Autodesk Inventor part; units mm, degrees
ref_plane "YZ Plane" through (0, 0, 0) normal (1, 0, 0) x (0, 1, 0)
ref_plane "XZ Plane" through (0, 0, 0) normal (0, 1, 0) x (-1, 0, 0)
ref_plane "XY Plane" through (0, 0, 0) normal (0, 0, 1) x (1, 0, 0)
sketch "Sketch1" plane through (0, 0, 0) normal (1, 0, 0) x (0, 1, 0)
  line L0 (9.0933, 11.7239) -> (-29.0067, 11.7239)
  line L1 (-29.0067, 11.7239) -> (-29.0067, -26.3761)
  line L2 (-29.0067, -26.3761) -> (9.0933, -26.3761)
  line L3 (9.0933, -26.3761) -> (9.0933, 11.7239)
  circle A0 centre (-9.9567, -7.3261) radius 6.35
  point P0 (0, 0)
  dimension "d0" = 38.1
  dimension "d1" = 38.1
  dimension "d2" = 12.7
  dimension "d3" = 19.05
  dimension "d4" = 19.05
extrude "Extrusion1" add sketch "Sketch1" along normal blind 25.4 contours L3 L2 L1 L0 | A0
sketch "Sketch2" plane through (25.4, 0, 0) normal (1, 0, 0) x (0, 0, -1)
  circle A0 centre (7.3261, -9.9567) radius 6.35
  line L0 (-11.7239, 9.0933) -> (-11.7239, -29.0067)
  line L1 (26.3761, 9.0933) -> (-11.7239, 9.0933)
  point P0 (0, 0)
  dimension "d7" = 12.7
  dimension "d8" = 19.05
  dimension "d9" = 19.05
extrude "Extrusion2" add sketch "Sketch2" along normal blind 88.9
sketch "Sketch3" plane through (114.3, -9.9567, -7.3261) normal (1, 0, 0) x (0, 0, -1)
  line L0 (-18.9201, 19.115) -> (19.1799, 19.115)
  line L1 (19.1799, 19.115) -> (19.1799, -18.985)
  line L2 (19.1799, -18.985) -> (-18.9201, -18.985)
  line L3 (-18.9201, -18.985) -> (-18.9201, 19.115)
  point P0 (-7.3261, 9.9567)
  dimension "d12" = 38.1
  dimension "d13" = 38.1
extrude "Extrusion3" add sketch "Sketch3" along normal blind 25.4
properties part number "belt axle"
Work out the finished part from the listing and answer in its coordinate system (mm). A direction names the side the tool comes from. Round coordinates to 2 decimals unless told otherwise and drop trailing zeros. Write each loop counter-clockwise with the first axis right and the second up, starting at its lowest first coordinate (ties: lowest second). Pieces come first, ordered by that corner, then holes.
1) A cutting plane is placed at A-A (z = -19). Give the vertices of the cut face in (x, y), plus the area to 3 significant figures.
2) A tool of negligible diameter and unlimited length cuts with its end or side. For faces 1 (the flat face through (13, -10, -26.376)), 2 (the flat face through (127, 9.158, -7)), 3 (the flat face through (25.4, -19, -7)), 4 (the flat face through (127, -10, 11.594)), from which of +Z, -Z, +X, -X, +Y, -Y can it reach the whole face along a straight path? Write none if from no direction.
3) The mould has two halves that part along X. Classify faces 5 (the flat face through (114.3, -1, -7)), 6 (the flat face through (139.7, -10, -7)), 7 (the flat face through (127, -10, -26.506)): pulls with the +X half, pulls with the -X half, needs draft (parallel to the pull), parting line crosses it, or undercut.
4) A cutting plane is placed at B-B (y = 3.5). Give the vertices of the cut face in (x, z).
5) Straight lines are drawn through the part: line 1 (X direction, y = -24, z = -5.5); line 2 (Z direction, x = 6, y = 4.5); line 3 (Z direction, x = 119, y = -9.5). For each, find the intervals that lie inside material, in ascending order.
6) Given pin 1 Ø12.5 at (x, y) = (122, -0.5) entering from +Z; pin 2 Ø20.5 at (x, z) = (127.5, 1) entering from -Y; pin 3 Ø7.5 at (x, y) = (17, -2.5) entering from -Z, each flat-ended and moving along its own axis, determine where each tip first touches the part or whether it passes through.
7) A cutting plane is placed at D-D (z = -5). Give the vertices of the cut face in (x, y), plus the area to 3 significant figures.
8) A cutting plane is placed at C-C (y = -7.5). Give the vertices of the cut face in (x, z), plus the area to 3 significant figures.
Completed:
1. outline: (0, -29.01) - (25.4, -29.01) - (25.4, 9.09) - (0, 9.09) - close; (114.3, -28.94) - (139.7, -28.94) - (139.7, 9.16) - (114.3, 9.16) - close
1. area: 1,940 mm2
2. face 1: -Z, -X, +Y, -Y
2. face 2: +Z, -Z, +X, -X, +Y
2. face 3: none
2. face 4: +Z, +X, +Y, -Y
3. face 5: undercut
3. face 6: pulls with the +X half
3. face 7: needs draft
4. outline: (0, -26.38) - (25.4, -26.38) - (25.4, 11.72) - (0, 11.72) - close; (114.3, -26.51) - (139.7, -26.51) - (139.7, 11.59) - (114.3, 11.59) - close
5. line 1: x = 0 to 25.4, 114.3 to 139.7
5. line 2: z = -26.38 to 11.72
5. line 3: z = -26.51 to 11.59
6. pin 1: stops at z = 11.59
6. pin 2: stops at y = -28.94
6. pin 3: stops at z = -26.38
7. outline: (0, -29.01) - (25.4, -29.01) - (25.4, -15.87) - (114.3, -15.87) - (114.3, -28.94) - (139.7, -28.94) - (139.7, 9.16) - (114.3, 9.16) - (114.3, -4.05) - (25.4, -4.05) - (25.4, 9.09) - (0, 9.09) - close
7. area: 2,990 mm2
8. outline: (0, -26.38) - (25.4, -26.38) - (25.4, -13.18) - (114.3, -13.18) - (114.3, -26.51) - (139.7, -26.51) - (139.7, 11.59) - (114.3, 11.59) - (114.3, -1.47) - (25.4, -1.47) - (25.4, 11.72) - (0, 11.72) - close
8. area: 2,980 mm2
